from build123d import *

# Parameters (mm, degrees)
BOSS_EXTRUDE1_DEPTH = 10
SKETCH2_W           = 30
SKETCH2_H           = 25
BOSS_EXTRUDE2_DEPTH = 5
BOSS_EXTRUDE3_DEPTH = 5


with BuildPart() as part:
    # Sketch1 → Boss-Extrude1 (new body)
    with BuildSketch(Plane(origin=(0, 0, 0), x_dir=(0, 0, -1), z_dir=(1, 0, 0))):
        Polygon((0, 0), (-10, 0), (-10, -20), (-30, -20), (-30, -25), (-10, -25), (-10, -38), (0, -38), align=None)
    extrude(amount=BOSS_EXTRUDE1_DEPTH)

    # Sketch2 → Boss-Extrude2 (add)
    with BuildSketch(Plane.ZY):
        with Locations((15, -12.5)):
            Rectangle(SKETCH2_W, SKETCH2_H)
    extrude(amount=BOSS_EXTRUDE2_DEPTH)

    # Sketch3 → Boss-Extrude3 (add)
    with BuildSketch(Plane(origin=(10, 0, 0), x_dir=(0, 0, -1), z_dir=(1, 0, 0))):
        Polygon((-10, 0), (-10, -20), (-30, -20), (-30, -25), (-10, -25), (0, -25), (0, 0), align=None)
    extrude(amount=BOSS_EXTRUDE3_DEPTH)


solid = part.part
For this review, take the finished solid that the model builds, in its own axes (mm). A direction names the side the tool comes from. Round coordinates to 2 decimals unless told otherwise and drop trailing zeros. Loops run counter-clockwise (first coordinate to the right, second up) from the corner with the lowest first, then second, coordinate; pieces in that order, holes last. Notation, with made-up numbers: (25.5, 51) - (34.5, 51) arc R20 cw to (34.5, 82) - close; hole circle Ø9 at (43, -17). An arc over 180 degrees is marked (long way). One line per item, written item: value. Start each with the question number.
Item 1: For faces 1 (the flat face through (10, -31, 5)), 2 (the flat face through (0, -31, 5)), 3 (the flat face through (0, -10, 20)), 4 (the flat face through (5, -31, 10)), list the 3-axis set-ups (+Z, -Z, +X, -X, +Y, -Y) from which the entire face can be reached by the end or side of a thin tool; tool diameter is ignored.
Item 2: For L1, parallel to X at y = -7, z = 16; L2, parallel to Y at x = 13.75, z = 22.5; L3, parallel to Y at x = -1.75, z = 16, list the stretches that pass through material, from the lowest coordinate up.
Item 3: Clearance check with flat-ended pins moving along their axes: pin 1 Ø3 at (y, z) = (-29, 4) entering from -X; pin 2 Ø8 at (x, y) = (8, -10.5) entering from -Z; pin 3 Ø7.5 at (x, z) = (4.5, 16.5) entering from +Y; pin 4 Ø8 at (x, y) = (7, -29.5) entering from +Z. State where each tip first meets the part, or that it passes through.
Item 4: Take a section at C-C (y = -28). Give the boundary of the cut face in (x, z).
Item 5: Take a section at D-D (x = 13.5). Give the boundary of the cut face in (y, z).
Item 6: Take a section at A-A (z = 2.75). Give the boundary of the cut face in (x, y).
Item 7: Take a section at B-B (x = 4.25). Give the boundary of the cut face in (y, z).
Answer below:
1. face 1: +Z, -Z, +X, -Y
1. face 2: +Z, -Z, -X, -Y
1. face 3: +Z, +X, +Y
1. face 4: +Z, +X, -X, -Y
2. L1: x = -5 to 0
2. L2: y = -25 to -20
2. L3: y = -25 to 0
3. pin 1: stops at x = 0
3. pin 2: stops at z = 0
3. pin 3: stops at y = -20
3. pin 4: stops at z = 10
4. outline: (0, 0) - (10, 0) - (10, 10) - (0, 10) - close
5. outline: (-25, 0) - (0, 0) - (0, 10) - (-20, 10) - (-20, 30) - (-25, 30) - close
6. outline: (-5, -25) - (0, -25) - (0, -38) - (10, -38) - (10, -25) - (15, -25) - (15, 0) - (-5, 0) - close
7. outline: (-38, 0) - (0, 0) - (0, 10) - (-20, 10) - (-20, 30) - (-25, 30) - (-25, 10) - (-38, 10) - close
